The model under review builds one solid part; all positions refer to its coordinate system, in mm. A direction names the side the tool comes from. Give positions to 0.01 mm unless a question says otherwise; leave off trailing zeros. Write each loop counter-clockwise with the first axis right and the second up, starting at its lowest first coordinate (ties: lowest second). Pieces come first, ordered by that corner, then holes. Notation, with made-up numbers: M -7.5,15.25 L 29.5,15.25 A30 cw 29.5,52.25 Z; hole C 13,-13 d5. An arc over 180 degrees is marked long. Write item = value, one per line. Start each with the question number.
Autodesk Inventor part; units mm, degrees
ref_plane "YZ Plane" through (0, 0, 0) normal (1, 0, 0) x (0, 1, 0)
ref_plane "XZ Plane" through (0, 0, 0) normal (0, 1, 0) x (-1, 0, 0)
ref_plane "XY Plane" through (0, 0, 0) normal (0, 0, 1) x (1, 0, 0)
sketch "Sketch1" plane through (0, 0, 0) normal (0, 0, 1) x (1, 0, 0)
  arc A0 (3.487, 25.0215) -> (1.7914, 25.1997) centre (0, 0) ccw
  arc A1 (5.6634, 19.703) -> (-1.4432, 20.4499) centre (0, 0) ccw
  arc A2 (164.4584, 30.6266) -> (162.8369, 30.0997) centre (171.45, 6.35) ccw
  arc A3 (168.6099, 26.6531) -> (161.8138, 24.4449) centre (171.45, 6.35) ccw
  arc A4 (172.385, -18.896) -> (170.515, 31.596) centre (171.45, 6.35) ccw
  arc A5 (172.2088, -14.1368) -> (170.6912, 26.8368) centre (171.45, 6.35) ccw
  arc A6 (-0.935, 25.246) -> (0.935, -25.246) centre (0, 0) ccw
  arc A7 (-0.7588, 20.4868) -> (0.7588, -20.4868) centre (0, 0) ccw
  line L0 (-0.935, 25.246) -> (170.515, 31.596)
  line L1 (0.935, -25.246) -> (172.385, -18.896)
  line L2 (-0.7588, 20.4868) -> (170.6912, 26.8368)
  line L3 (0.7588, -20.4868) -> (172.2088, -14.1368)
  point P0 (0, 0)
extrude "Extrusion1" add sketch "Sketch1" along normal blind 3.175
properties part number "Chain"
Item 1: The part is to be moulded in two halves that separate along X. For faces 3 (the flat face through (85, 24, 3.175)), 4 (the flat face through (83.766, 23.617, 1.565)), 5 (the flat face through (85.46, -22.115, 1.565)), say which applies: released by +X, released by -X, zero draft, split by the parting line, or undercut.
Item 2: We need section C-C, the plane y = 8. Write out the cut boundary in (x, z) (1 decimal), and give its area (3 significant figures).
Item 3: Clearance check with flat-ended pins moving along their axes: P1, Ø1.5, axis at y = -11, z = 1.5, coming from the +X side; P2, Ø1.5, axis at y = -10, z = 2, coming from the -X side; P3, Ø10, axis at x = 153.5, y = -9.5, coming from the -Z side; P4, Ø1, axis at x = 128, z = 2, coming from the -Y side. State where each tip first meets the part, or that it passes through.
Item 4: We need section A-A, the plane z = 1.8. Write out the cut boundary in (x, y) (3 decimals).
Item 5: To check wall thickness, follow probe 1 along Y at (x, z) = (172, 1.8); probe 2 along X at (y, z) = (4.5, 1.75); probe 3 along Y at (x, z) = (98, 0.8). State the ranges of each line that lie inside material, in increasing order. Write a range as [from, to].
Item 6: For faces 1 (the cylindrical face through (-20.442, -1.546, 1.565)), 2 (the flat face through (85, 24, 0)), list the 3-axis set-ups (+Z, -Z, +X, -X, +Y, -Y) from which the entire face can be reached by the end or side of a thin tool; tool diameter is ignored.
Item 7: We need section B-B, the plane x = 74. Write out the cut boundary in (y, z) (3 decimals), and give its area (3 significant figures).
Worked out:
q1.face_3 = zero draft
q1.face_4 = undercut
q1.face_5 = released by +X
q2.outline = M -24,0 L -18.9,0 L -18.9,3.2 L -24,3.2 Z; M 191.9,0 L 196.7,0 L 196.7,3.2 L 191.9,3.2 Z
q2.area = 31.3 mm²
q3.P1 = 190.49
q3.P2 = -23.51
q3.P3 = through
q3.P4 = -20.56
q4.outline = M -0.935,25.246 A25.263 ccw 0.935,-25.246 L 172.385,-18.896 A25.263 ccw 170.515,31.596 Z; hole M -1.443,20.45 A20.501 ccw 0.759,-20.487 L 172.209,-14.137 A20.501 ccw 170.691,26.837 L -0.759,20.487 A20.5 ccw Z
q5.probe_1 = [-18.91, -14.14], [26.84, 31.61]
q5.probe_2 = [-24.86, -20], [191.87, 196.65]
q5.probe_3 = [-21.65, -16.89], [24.14, 28.91]
q6.face_1 = +Z, -Z
q6.face_2 = -Z, +X, -X, +Y, -Y
q7.outline = M -22.54,0 L -17.774,0 L -17.774,3.175 L -22.54,3.175 Z; M 23.256,0 L 28.021,0 L 28.021,3.175 L 23.256,3.175 Z
q7.area = 30.3 mm²
